```python
from build123d import *
from build123d import SkipClean  # not in build123d's __all__

# Parameters (mm, degrees)
F1_DEPTH = 6


with BuildPart() as f1:
    # F0 (on Front) → F1 (new body)
    with BuildSketch(Plane.XZ):
        with BuildLine():
            Line((-57.5, 0), (0, 0))
            Line((0, 0), (0, 20.925))
            ThreePointArc((0, 20.925), (-10.075, 31), (0, 41.075))
            Line((0, 41.075), (0, 53))
            Line((0, 53), (-62.5, 53))
            Line((-62.5, 53), (-62.5, 3))
            Line((-62.5, 3), (-57.5, 3))
            Line((-57.5, 3), (-57.5, 0))
        make_face()
    extrude(amount=F1_DEPTH)

    # F2: F1 across face


with BuildPart() as f1_1:
    add(f1.part, clean=False)
    with SkipClean():  # cleaning this boolean's faces spoils the solid; the shape is the same uncleaned
        add(f1.part.mirror(Plane(origin=(0, -3, 47.0375), x_dir=(0, 1, 0), z_dir=(1, 0, 0))), clean=False)


solid = f1_1.part
```
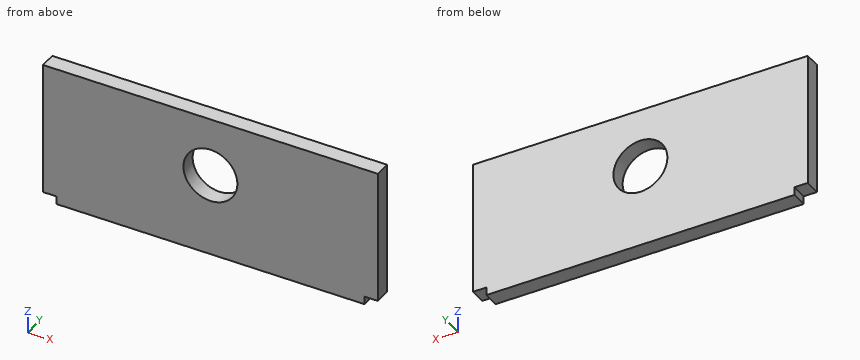
Check sheet for the modelled part. Datum: model origin and axes. Units: mm. Round coordinates to 2 decimals unless told otherwise and drop trailing zeros. Write each loop counter-clockwise with the first axis right and the second up, starting at its lowest first coordinate (ties: lowest second). Pieces come first, ordered by that corner, then holes. Notation, with made-up numbers: (70, -31) -> (111, -31) arc R29 ccw to (111, -6) -> close; hole circle Ø10 at (78.5, 59.25). An arc over 180 degrees is marked (long way). One line per question, with ' | ' between items. Start each with the question number.
1. Depth check by flat-ended pin: pin 1 (12 mm diameter, centred on x = 0, z = 31, fed in from -Y); pin 2 (3.5 mm diameter, centred on y = -4.5, z = 1, fed in from +X); pin 3 (1.5 mm diameter, centred on x = -60, y = -4, fed in from -Z). Enter the tip coordinate at first touch or a pass-through.
2. Sectioned sample at B-B, the plane z = 31. Record the cut outline in (x, y) (3 decimals).
3. Scan lines: line 1 along X through (y, z) = (-4.45, 31) (3 decimals); line 2 along Z through (x, y) = (0, -3.3) (3 decimals); line 3 along Z through (x, y) = (2, -1.95). Record each from-to range of solid material in increasing order. Write a range as from..to.
4. Sectioned sample at C-C, the plane y = -2.1. Record the cut outline in (x, z) (3 decimals).
5. Sectioned sample at A-A, the plane x = 0. Record the cut outline in (y, z) (3 decimals), then the cut area to 3 significant figures.
Taken from the geometry:
1) pin 1: passes through | pin 2: stops at x = 57.5 | pin 3: stops at z = 3
2) outline: (-62.5, -6) -> (-10.075, -6) -> (-10.075, 0) -> (-62.5, 0) -> close; (10.075, -6) -> (62.5, -6) -> (62.5, 0) -> (10.075, 0) -> close
3) line 1: x = -62.5..-10.075, 10.075..62.5 | line 2: z = 0..20.925, 41.075..53 | line 3: z = 0..21.13, 40.87..53
4) outline: (-62.5, 3) -> (-57.5, 3) -> (-57.5, 0) -> (57.5, 0) -> (57.5, 3) -> (62.5, 3) -> (62.5, 53) -> (-62.5, 53) -> close; hole circle Ø20.15 at (0, 31)
5) outline: (-6, 0) -> (0, 0) -> (0, 20.925) -> (-6, 20.925) -> close; (-6, 41.075) -> (0, 41.075) -> (0, 53) -> (-6, 53) -> close | area: 197 mm^2
